Here's the drawing with two shaded views (mm, measured from the low corner). I have some questions. A direction names the side the tool comes from. Coordinates: 2 decimals unless noted, no trailing zeros. Write each loop counter-clockwise with the first axis right and the second up, starting at its lowest first coordinate (ties: lowest second). Pieces come first, ordered by that corner, then holes.
Item 1: For P1, Ø1.5, axis at x = 59.5, z = 67.5, coming from the +Y side (1 decimal); P2, Ø6, axis at x = 51.5, y = 81, coming from the +Z side, each with a flat end and sliding along its axis, tell me the tip position at first contact or that it passes through.
Item 2: Which directions (+Z, -Z, +X, -X, +Y, -Y) give clear straight access to the entire face, cutting with the end or side of a thin tool? Please do the marked faces 1 and 2.
Item 3: If I drill on probe 1 along Z at (x, y) = (25.5, 76.5) (1 decimal); probe 2 along Z at (x, y) = (78.5, 84); probe 3 along Z at (x, y) = (14.5, 30) (1 decimal), over which ranges is the centre line in solid material (lowest first)?
Item 4: I want a section at D-D on x = 77.5. Please give me the cut outline in (y, z), then the cut area to 3 significant figures.
Item 5: Thinking about a two-plate mould opening in Z: for the marked faces 3, 4 and 5, which applies, +Z half, -Z half, draft (parallel to the pull), parting line (faces both ways), or undercut?
Item 6: I want a section at A-A on x = 44. Please give me the cut outline in (y, z).
Item 7: I want a section at C-C on z = 31. Please give me the cut outline in (x, y), then the cut area to 3 significant figures.
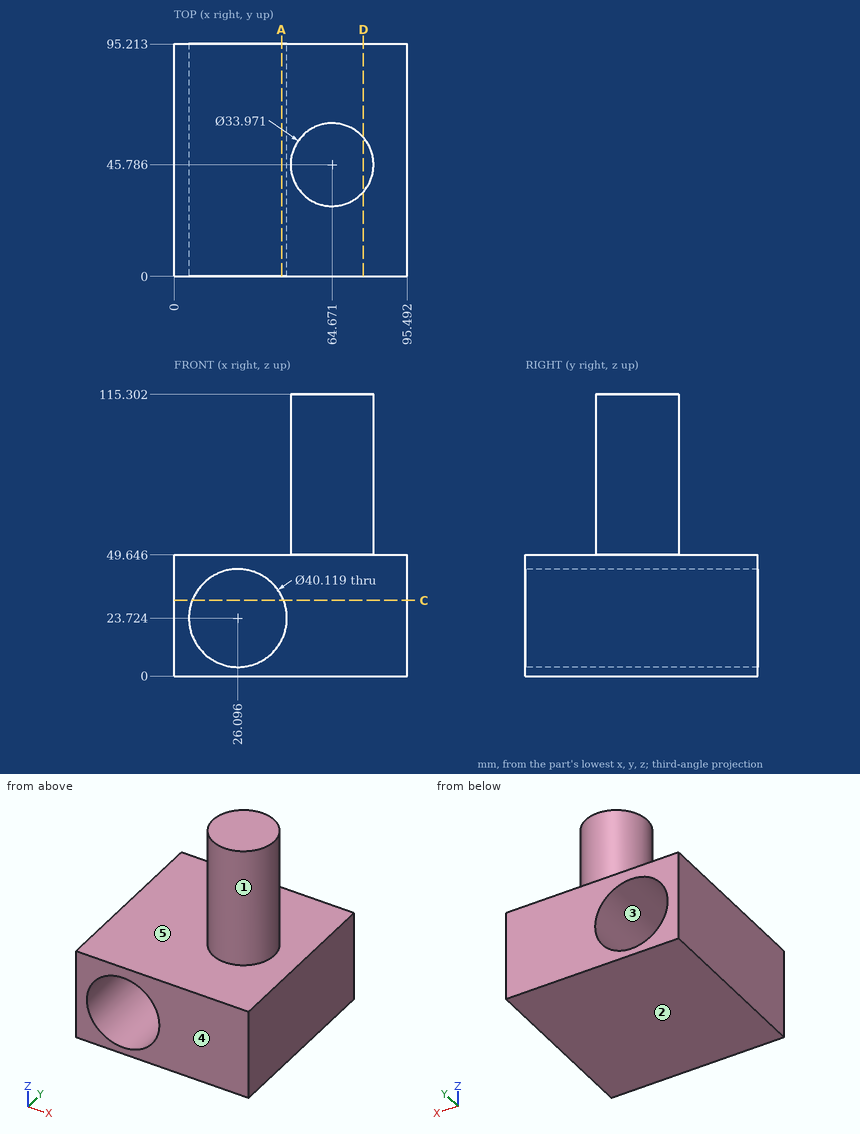
Response values:
1. P1: stops at y = 62.2
1. P2: stops at z = 49.65
2. face 1: +Z
2. face 2: -Z, +X, -X, +Y, -Y
3. probe 1: z = 0 to 3.7, 43.8 to 49.6
3. probe 2: z = 0 to 49.65
3. probe 3: z = 0 to 7.4, 40.1 to 49.6
4. outline: (0, 0) - (95.21, 0) - (95.21, 49.65) - (56.92, 49.65) - (56.92, 115.3) - (34.65, 115.3) - (34.65, 49.65) - (0, 49.65) - close
4. area: 6,190 mm2
5. face 3: undercut
5. face 4: draft
5. face 5: +Z half
6. outline: (0, 0) - (95.21, 0) - (95.21, 14.68) - (0, 14.68) - close; (0, 32.77) - (95.21, 32.77) - (95.21, 49.65) - (0, 49.65) - close
7. outline: (0, 0) - (7.4, 0) - (7.4, 95.21) - (0, 95.21) - close; (44.79, 0) - (95.49, 0) - (95.49, 95.21) - (44.79, 95.21) - close
7. area: 5,530 mm2
